Print and shaded views of the part. All mm, measured from the part's lowest x, y and z. Give positions to 0.01 mm unless a question says otherwise; leave off trailing zeros. Order: outer loops, then holes, each group sorted by start corner. A loop starts at its lowest first (then second) coordinate and runs counter-clockwise, first axis right, second up. Notation, with made-up numbers: (-3.5, 64) - (51.5, 64) arc R24 cw to (51.5, 99) - close; hole circle Ø3 at (89.5, 57). An arc over 180 degrees is marked (long way). Answer in a Markdown table with one row per item.
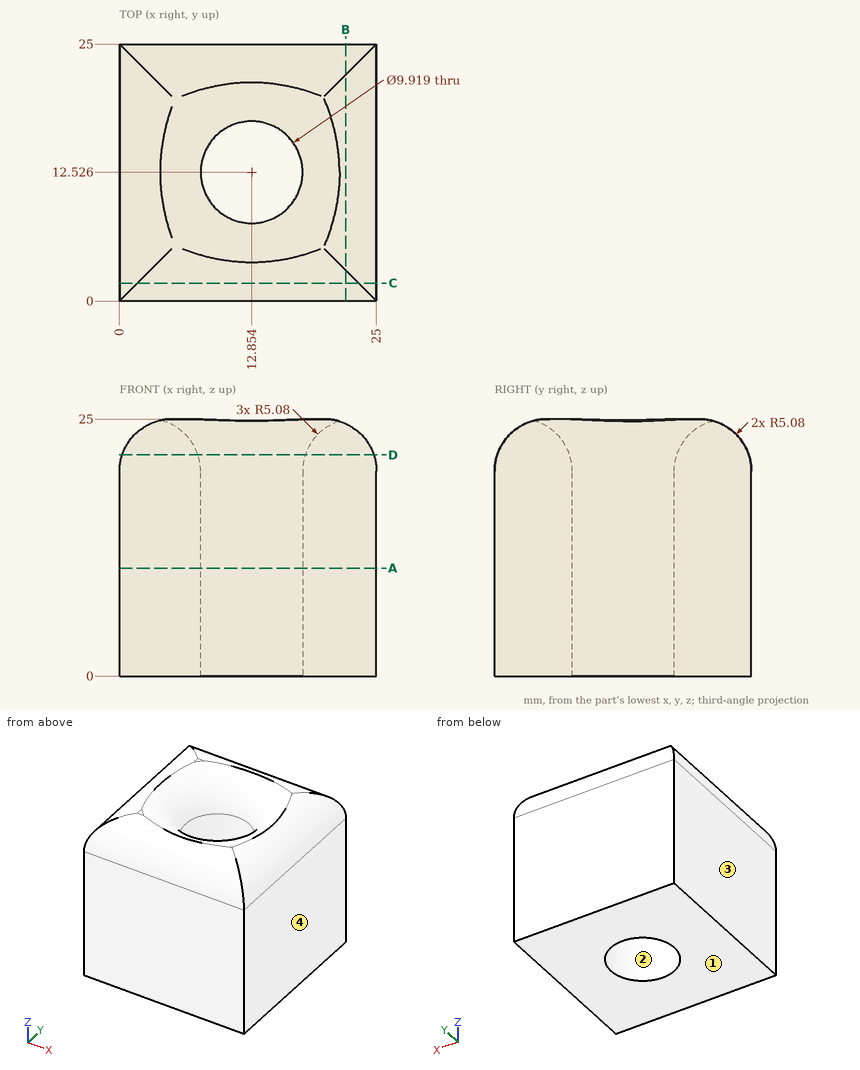
1. Two-plate mould, pull along X, no slides. Class the marked faces 1, 2, 3 and 4: +X half, -X half, draft (parallel to the pull), parting line (faces both ways), or undercut.
Check result:
| item | result |
|---|---|
| face 1 | draft |
| face 2 | undercut |
| face 3 | -X half |
| face 4 | +X half |
2. Cut at D-D on z = 21.5. Write the cut outline in (x, y) (1 decimal), and give its area (3 significant figures).
Check result:
| item | result |
|---|---|
| outline | (0.3, 0.3) - (24.7, 0.3) - (24.7, 24.7) - (0.3, 24.7) - close; hole circle Ø10.4 at (12.9, 12.5) |
| area | 515 mm² |
3. Probe line 1 (X direction, y = 12.5, z = 19.75) (1 decimal); line 2 (X direction, y = 8.75, z = 17.75); line 3 (Y direction, x = 15, z = 7.5) (1 decimal). List the from-to ranges inside material, lowest first.
Check result:
| item | result |
|---|---|
| line 1 | x = 0 to 7.9, 17.8 to 25 |
| line 2 | x = 0 to 9.64, 16.07 to 25 |
| line 3 | y = 0 to 8.1, 17 to 25 |
4. Cut at C-C on y = 1.75. Write the cut outline in (x, z).
Check result:
| item | result |
|---|---|
| outline | (0, 0) - (25, 0) - (25, 19.92) arc R5.08 ccw to (23.25, 23.76) - (1.75, 23.76) arc R5.08 ccw to (0, 19.92) - close |
5. Cut at B-B on x = 22. Write the cut outline in (y, z) (1 decimal).
Check result:
| item | result |
|---|---|
| outline | (0, 0) - (25, 0) - (25, 19.9) arc R5.1 ccw to (22, 24.6) - (3, 24.6) arc R5.1 ccw to (0, 19.9) - close |
6. Cut at A-A on z = 10.5. Write the cut outline in (x, y) (1 decimal), and give its area (3 significant figures).
Check result:
| item | result |
|---|---|
| outline | (0, 0) - (25, 0) - (25, 25) - (0, 25) - close; hole circle Ø9.9 at (12.9, 12.5) |
| area | 548 mm² |
7. Drop a flat-ended pin along its axis: P1, Ø4, axis at x = 16.5, y = 15, coming from the +Z side. Give the stop position or say it passes through.
Check result:
| item | result |
|---|---|
| P1 | stops at z = 23.47 |
